from build123d import *

# Parameters (mm, degrees)
SKETCH_R     = 15
PAD_DEPTH    = 15
SKETCH002_R  = 5
PAD001_DEPTH = 20


with BuildPart() as part:
    # Sketch → Pad (new body, symmetric)
    with BuildSketch(Plane.XY):
        Circle(SKETCH_R)
    extrude(amount=PAD_DEPTH, both=True)

    # Sketch002 → Pad001 (join, symmetric)
    with BuildSketch(Plane.XY):
        Circle(SKETCH002_R)
    extrude(amount=PAD001_DEPTH, both=True)


solid = part.part
Read the model definition and answer for the solid it produces. Units are mm, in the model's axes. A direction names the side the tool comes from. Round coordinates to 2 decimals unless told otherwise and drop trailing zeros. Loops run counter-clockwise (first coordinate to the right, second up) from the corner with the lowest first, then second, coordinate; pieces in that order, holes last. Notation, with made-up numbers: (63.5, 60.5) - (81.5, 60.5) arc R27 ccw to (81.5, 90.5) - close; hole circle Ø11 at (-24, 12.5). An arc over 180 degrees is marked (long way). One line per question, with ' | ' between items. Start each with the question number.
Q1. Flat-ended cylindrical pins translate along their axes: pin 1 (2 mm diameter, centred on y = 7, z = 1, fed in from +X); pin 2 (1.5 mm diameter, centred on y = 11.5, z = -16, fed in from -X); pin 3 (3 mm diameter, centred on x = 9, y = -11.5, fed in from +Z); pin 4 (12 mm diameter, centred on y = -9, z = 11, fed in from +X). Find the tip coordinate at first contact, or state that the pin passes through.
Q2. Find the intervals of material crossed by L1, parallel to Z at x = 4, y = 12.5; L2, parallel to X at y = -0.75, z = 13; L3, parallel to X at y = -6.25, z = -0.5, in increasing order.
Q3. Section D-D on z = 16 is taken. Give the vertices of the cut face in (x, y).
Q4. Section A-A on y = 0 is taken. Give the vertices of the cut face in (x, z), plus the area to 3 significant figures.
Q5. Section C-C on z = -13 is taken. Give the vertices of the cut face in (x, y).
Q6. For faces 1 (the cylindrical face through (-1.08, -4.88, 17.54)), 2 (the flat face through (0, 0, 20)), 3 (the cylindrical face through (-1.08, -4.88, -17.46)), determine the directions among +Z, -Z, +X, -X, +Y, -Y from which every point of the face is accessible in a straight line to the end or side of a thin tool.
Established:
1) pin 1: x = 13.75 | pin 2: through | pin 3: z = 15 | pin 4: x = 14.7
2) L1: -15 to 15 | L2: -14.98 to 14.98 | L3: -13.64 to 13.64
3) outline: circle Ø10 at (0, 0)
4) outline: (-15, -15) - (-5, -15) - (-5, -20) - (5, -20) - (5, -15) - (15, -15) - (15, 15) - (5, 15) - (5, 20) - (-5, 20) - (-5, 15) - (-15, 15) - close | area: 1,000 mm²
5) outline: circle Ø30 at (0, 0)
6) face 1: +Z | face 2: +Z, +X, -X, +Y, -Y | face 3: -Z
